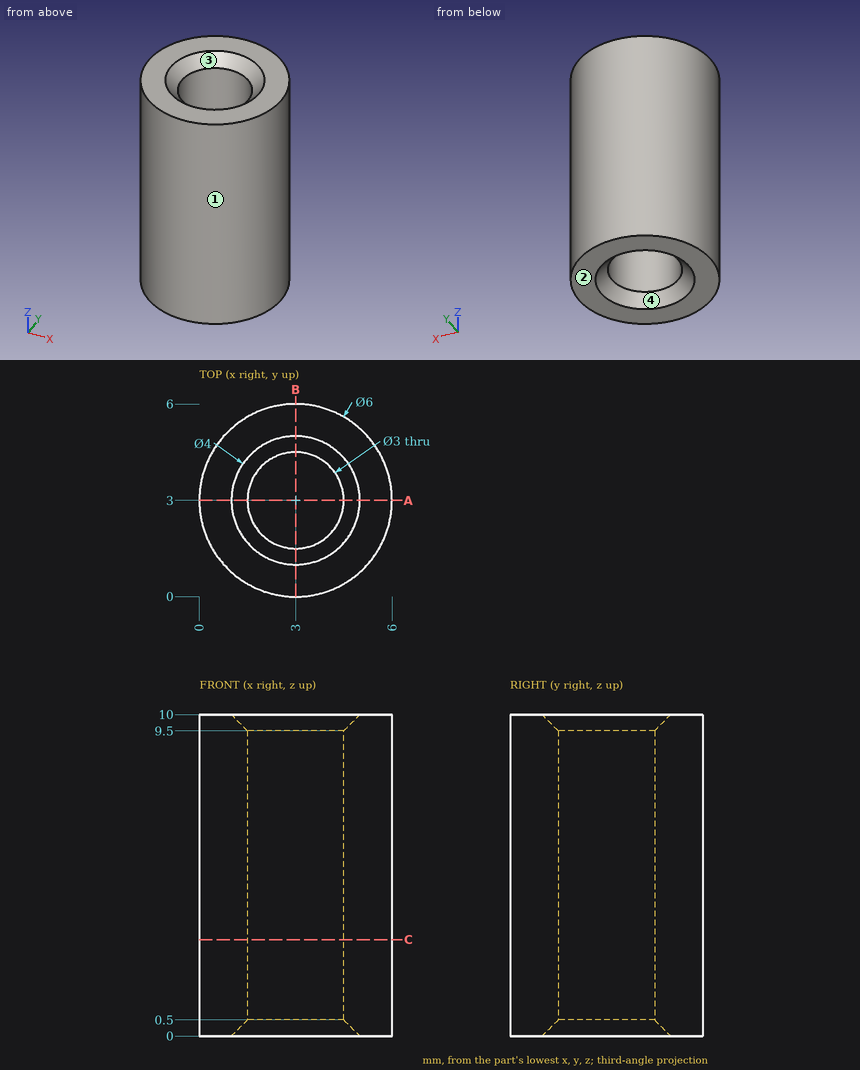
Answer from the drawing. Dimensions are ordinates in mm from the lowest x, y and z of the part. Coordinates: 2 decimals unless noted, no trailing zeros. Loops run counter-clockwise (first coordinate to the right, second up) from the corner with the lowest first, then second, coordinate; pieces in that order, holes last.
Q1. The part is cut by section C-C on z = 3. Write down the section's boundary in (x, y), and give its area (3 significant figures).
Q2. Consider probe 1 along Y at (x, z) = (3, 3); probe 2 along Y at (x, z) = (3.8, 4.75); probe 3 along X at (y, z) = (1.85, 7.25). Determine where each line is inside the solid, lowest interval first.
Q3. The part is cut by section A-A on y = 3. Write down the section's boundary in (x, z).
Q4. The mould has two halves that part along Y. Classify the marked faces 1, 2, 3 and 4: +Y half, -Y half, draft (parallel to the pull), parting line (faces both ways), or undercut.
Q5. This flat-tipped pin is pushed along its axis until it touches: pin 1 Ø1 at (y, z) = (2, 5.5) entering from +X. Where does it stop, or does it pass through?
Results below:
1. outline: circle Ø6 at (3, 3); hole circle Ø3 at (3, 3)
1. area: 21.2 mm2
2. probe 1: y = 0 to 1.5, 4.5 to 6
2. probe 2: y = 0.11 to 1.73, 4.27 to 5.89
2. probe 3: x = 0.23 to 2.04, 3.96 to 5.77
3. outline: (0, 0) - (1, 0) - (1.5, 0.5) - (1.5, 9.5) - (1, 10) - (0, 10) - close; (4.5, 0.5) - (5, 0) - (6, 0) - (6, 10) - (5, 10) - (4.5, 9.5) - close
4. face 1: parting line
4. face 2: draft
4. face 3: undercut
4. face 4: undercut
5. pin 1: stops at x = 5.96
